Source: CAD feature listing. Evaluate the final solid. Frame: model axes, mm. Face numbers are marked on the shaded views. A direction names the side the tool comes from. Coordinates: 2 decimals unless noted, no trailing zeros. Write each loop counter-clockwise with the first axis right and the second up, starting at its lowest first coordinate (ties: lowest second). Pieces come first, ordered by that corner, then holes. Notation, with made-up numbers: (69.25, 65.25) - (86.25, 65.25) arc R17 cw to (86.25, 92.25) - close; hole circle Ø6 at (-16, 87). An arc over 180 degrees is marked (long way). One line per question, with ' | ' between items. Start each with the question number.
Q1. Cut plane C-C, the plane z = -25.4. Return loops of the section in (x, y) (3 decimals).
Q2. Contact query for flat-ended pins moving along their axis: P1, Ø12, axis at x = 14, z = -42, coming from the -Y side; P2, Ø12.5, axis at x = 17, y = 30.5, coming from the -Z side (3 decimals); P3, Ø5, axis at x = 12.7, y = 38.1, coming from the +Z side; P4, Ø1, axis at x = 12, z = -17.5, coming from the +Y side (3 decimals). Output: stop coordinate, or through.
Q3. Access query for the marked faces 1 and 2. Directions: +Z, -Z, +X, -X, +Y, -Y. A direction counts if a zero-diameter tool reaches every point of the face in a straight line with its end or side. Return the directions, or none.
Q4. Line query: line 1 (Y direction, x = 12.7, z = -1.85) (3 decimals); line 2 (X direction, y = 38, z = -1); line 3 (Y direction, x = 6.75, z = -18) (3 decimals). Output: solid intervals per line, ascending.
Q5. Cut plane D-D, the plane x = 21.5. Return loops of the section in (y, z) (3 decimals).
Q6. Cut plane B-B, the plane x = 12.7. Return loops of the section in (y, z) (3 decimals), plus the area to 3 significant figures.
Q7. Cut plane A-A, the plane y = 38.1. Return loops of the section in (x, z) (3 decimals), plus the area to 3 significant figures.
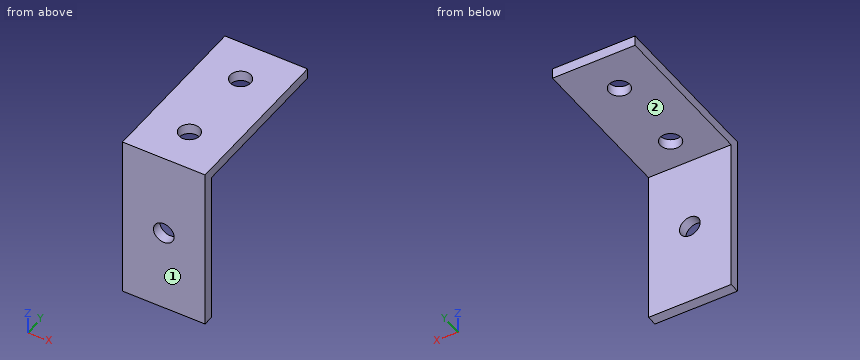
Autodesk Inventor part; units mm, degrees
ref_plane "YZ Plane" through (0, 0, 0) normal (1, 0, 0) x (0, 1, 0)
ref_plane "XZ Plane" through (0, 0, 0) normal (0, 1, 0) x (-1, 0, 0)
ref_plane "XY Plane" through (0, 0, 0) normal (0, 0, 1) x (1, 0, 0)
sketch "Sketch1" plane through (0, 0, 0) normal (1, 0, 0) x (0, 1, 0)
  line L0 (0, 0) -> (50.8, 0)
  line L1 (50.8, 0) -> (50.8, -3.175)
  line L2 (3.175, -50.8) -> (0, -50.8)
  line L3 (0, -50.8) -> (0, 0)
  line L4 (3.175, -50.8) -> (3.175, -3.175)
  line L5 (3.175, -3.175) -> (50.8, -3.175)
  dimension "d0" = 3.175
  dimension "d1" = 50.8
extrude "Extrusion1" add sketch "Sketch1" along normal blind 25.4
sketch "Sketch2" plane through (0, 3.175, -3.175) normal (0, 1, 0) x (1, 0, 0)
  line L0 (0, 47.625) -> (25.4, 47.625)
  line L1 (12.7, 47.625) -> (12.7, 11.1903) construction
  circle A0 centre (12.7, 22.225) radius 3.175
  line L2 (0, -3.175) -> (25.4, -3.175)
  dimension "d4" = 6.35
  dimension "d5" = 25.4
extrude "Extrusion2" cut sketch "Sketch2" against normal blind 3.175
sketch "Sketch4" plane through (0, 3.175, -3.175) normal (0, 0, -1) x (-1, 0, 0)
  line L0 (0, 47.625) -> (-25.4, 47.625)
  line L1 (-12.7, 47.625) -> (-12.7, 26.8905) construction
  circle A0 centre (-12.7, 34.925) radius 3.175
  circle A1 centre (-12.7, 9.525) radius 3.175
  line L2 (0, -3.175) -> (-25.4, -3.175)
  dimension "d8" = 6.35
  dimension "d9" = 12.7
  dimension "d10" = 38.1
extrude "Extrusion3" cut sketch "Sketch4" against normal blind 3.175
properties part number "Bracket"
Reply:
1) outline: (0, 0) - (9.525, 0) - (9.525, 3.175) - (0, 3.175) - close; (15.875, 0) - (25.4, 0) - (25.4, 3.175) - (15.875, 3.175) - close
2) P1: stops at y = 0 | P2: stops at z = -3.175 | P3: passes through | P4: stops at y = 3.175
3) face 1: +Z, -Z, +X, -X, -Y | face 2: -Z, +X, -X, +Y
4) line 1: y = 0 to 9.525, 15.875 to 34.925, 41.275 to 50.8 | line 2: x = 0 to 9.53, 15.87 to 25.4 | line 3: y = 0 to 3.175
5) outline: (0, -50.8) - (3.175, -50.8) - (3.175, -3.175) - (50.8, -3.175) - (50.8, 0) - (0, 0) - close
6) outline: (0, -50.8) - (3.175, -50.8) - (3.175, -28.575) - (0, -28.575) - close; (0, -22.225) - (3.175, -22.225) - (3.175, -3.175) - (9.525, -3.175) - (9.525, 0) - (0, 0) - close; (15.875, -3.175) - (34.925, -3.175) - (34.925, 0) - (15.875, 0) - close; (41.275, -3.175) - (50.8, -3.175) - (50.8, 0) - (41.275, 0) - close | area: 252 mm^2
7) outline: (0, -3.175) - (9.525, -3.175) - (9.525, 0) - (0, 0) - close; (15.875, -3.175) - (25.4, -3.175) - (25.4, 0) - (15.875, 0) - close | area: 60.5 mm^2
